Work out the finished part from the listing and answer in its coordinate system (mm). Coordinates: 2 decimals unless noted, no trailing zeros. Write each loop counter-clockwise with the first axis right and the second up, starting at its lowest first coordinate (ties: lowest second). Pieces come first, ordered by that corner, then holes. Notation, with made-up numbers: (39.5, 78.5) - (91.5, 78.5) arc R20 cw to (91.5, 89.5) - close; hole circle Ø11 at (73, 72). An arc over 180 degrees is marked (long way). Use one line per item in the form item = value. Start each with the question number.
Item 1: A cutting plane is placed at A-A (z = 1.7). Write down the section's boundary in (x, y), then the cut area to 3 significant figures.
Item 2: Consider probe 1 along Y at (x, z) = (29.5, 3.05); probe 2 along X at (y, z) = (-76, 0.65); probe 3 along Y at (x, z) = (-6, 3.35). Determine where each line is inside the solid, lowest interval first.
Item 3: Given pin 1 (2.5 mm diameter, centred on x = -4.5, y = -74.84, fed in from -Z), flat-ended and moving along its own axis, determine where the tip first touches the part or whether it passes through.
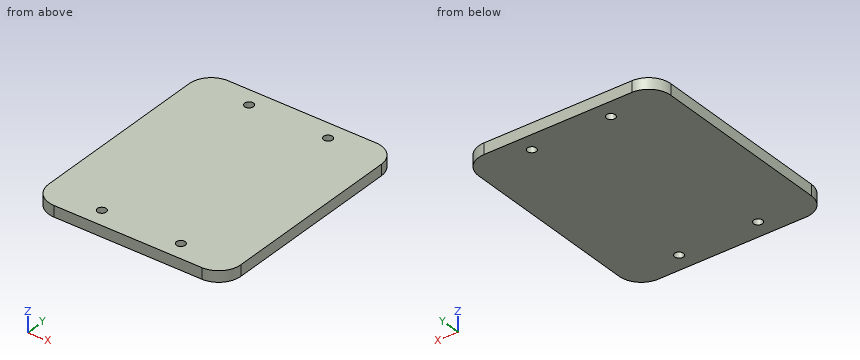
from build123d import *

# Parameters (mm, degrees)
CROQUIS1_W              = 87
CROQUIS1_H              = 103
CROQUIS1_R              = 2
SALIENTE_EXTRUIR1_DEPTH = 5
REDONDEO1_R             = 10


with BuildPart() as part:
    # Croquis1 → Saliente-Extruir1 (new body)
    with BuildSketch(Plane.XY):
        with Locations((13.390838462, -31.317238422)):
            Rectangle(CROQUIS1_W, CROQUIS1_H)
        with Locations((-4.499161538, 12.202761578)):
            Circle(CROQUIS1_R, mode=Mode.SUBTRACT)
        with Locations(Location((31.280838462, 12.202761578, 0), (0, 0, 180))):
            Circle(CROQUIS1_R, mode=Mode.SUBTRACT)
        with Locations((31.280838462, -74.837238422)):
            Circle(CROQUIS1_R, mode=Mode.SUBTRACT)
        with Locations(Location((-4.499161538, -74.837238422, 0), (0, 0, 180))):
            Circle(CROQUIS1_R, mode=Mode.SUBTRACT)
    extrude(amount=SALIENTE_EXTRUIR1_DEPTH)

    # Redondeo1
    redondeo1_edges = [part.edges().sort_by_distance(p)[0] for p in [
        (-30.109161538, 20.182761578, 2.5),
        (56.890838462, 20.182761578, 2.5),
        (56.890838462, -82.817238422, 2.5),
        (-30.109161538, -82.817238422, 2.5),
    ]]
    fillet(redondeo1_edges, radius=REDONDEO1_R)


solid = part.part
Answer:
q1.outline = (-30.11, -72.82) arc R10 ccw to (-20.11, -82.82) - (46.89, -82.82) arc R10 ccw to (56.89, -72.82) - (56.89, 10.18) arc R10 ccw to (46.89, 20.18) - (-20.11, 20.18) arc R10 ccw to (-30.11, 10.18) - close; hole circle Ø4 at (-4.5, -74.84); hole circle Ø4 at (-4.5, 12.2); hole circle Ø4 at (31.28, -74.84); hole circle Ø4 at (31.28, 12.2)
q1.area = 8,820 mm²
q2.probe_1 = -82.82 to -75.75, -73.93 to 11.29, 13.11 to 20.18
q2.probe_2 = -29.59 to -6.13, -2.87 to 29.65, 32.91 to 56.37
q2.probe_3 = -82.82 to -76.16, -73.52 to 10.88, 13.52 to 20.18
q3.pin_1 = through
